Solid Edge part; units mm, degrees
sketch "Sketch1" plane through (0, 0, 0) normal (0, 0, 1) x (1, 0, 0)
  line L0 (30, 10) -> (0, 10)
  line L1 (0, 10) -> (0, 0)
  line L2 (0, 0) -> (30, 0)
  line L3 (30, 0) -> (30, 10)
extrude "Protrusion1" add sketch "Sketch1" along normal blind 5
fillet "Round_1" radius 5 4 edges at (30, 0, 2.5) (30, 10, 2.5) (0, 10, 2.5) (0, 0, 2.5)
fillet "Round_2" radius 2 3 edges at (15, 10, 5) (0, 5, 5) (15, 0, 5)
sketch "Sketch2" plane through (15, 5, 0) normal (0, 0, -1) x (1, 0, 0)
  line L0 (10, 6) -> (-10, 6)
  arc A0 (-10, 6) -> (-10, -6) centre (-10, 0) ccw
  line L1 (-10, -6) -> (10, -6)
  arc A1 (10, -6) -> (10, 6) centre (10, 0) ccw
extrude "ExtrudedProtrusion_2" add sketch "Sketch2" along normal blind 1
properties material "ABS Plastic, high impact"
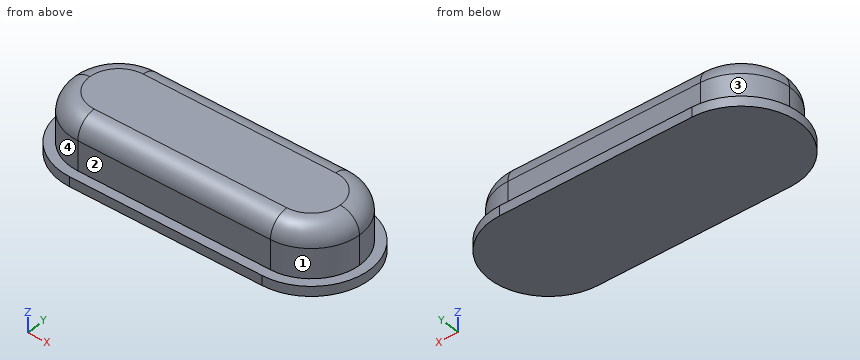
For this review, take the finished solid that the model builds, in its own axes (mm). Face numbers are marked on the shaded views. A direction names the side the tool comes from. Round coordinates to 2 decimals unless told otherwise and drop trailing zeros. Write each loop counter-clockwise with the first axis right and the second up, starting at its lowest first coordinate (ties: lowest second). Pieces come first, ordered by that corner, then holes. Notation, with made-up numbers: (42, 15.25) -> (83, 15.25) arc R31 cw to (83, 52.25) -> close; hole circle Ø9 at (34.5, 42.25). An arc over 180 degrees is marked (long way). Use one line per item in the form item = value.
Q1. To check wall thickness, follow probe 1 along Y at (x, z) = (6.5, 2); probe 2 along Z at (x, y) = (30.5, 6.75); probe 3 along X at (y, z) = (1, 0.15). State the ranges of each line that lie inside material, in increasing order. Write a range as from..to.
Resolved:
probe_1 = 0..10
probe_2 = -1..0
probe_3 = 2..28
Q2. Machinability: for the marked faces 1, 2, 3 and 4, which of the approach directions +Z, -Z, +X, -X, +Y, -Y give a long, thin tool a straight path to every point of the face, cutting with its end or side? Answer none if there is none.
Resolved:
face_1 = +Z, +X, -Y
face_2 = +Z, +X, -X, -Y
face_3 = +Z, -X, +Y
face_4 = +Z, -X, -Y
Q3. Clearance check with flat-ended pins moving along their axes: pin 1 Ø1.5 at (x, z) = (16.5, 1.5) entering from -Y; pin 2 Ø3.5 at (x, z) = (19.5, 2) entering from +Y; pin 3 Ø3 at (y, z) = (9, 2) entering from +X. State where each tip first meets the part, or that it passes through.
Resolved:
pin_1 = 0
pin_2 = 10
pin_3 = 29.33
Q4. Consider section D-D (z = -0.35). State the section outline as (x, y) points, then the cut area to 3 significant figures.
Resolved:
outline = (5, -1) -> (25, -1) arc R6 ccw to (25, 11) -> (5, 11) arc R6 ccw to start
area = 353 mm²
Q5. Consider section B-B (x = 7). State the section outline as (y, z) points, then the cut area to 3 significant figures.
Resolved:
outline = (-1, -1) -> (11, -1) -> (11, 0) -> (10, 0) -> (10, 3) arc R2 ccw to (8, 5) -> (2, 5) arc R2 ccw to (0, 3) -> (0, 0) -> (-1, 0) -> close
area = 60.3 mm²
